Here's how the part is built. I have some questions about the finished solid (model axes, mm). A direction names the side the tool comes from. Round coordinates to 2 decimals unless told otherwise and drop trailing zeros. Order: outer loops, then holes, each group sorted by start corner. A loop starts at its lowest first (then second) coordinate and runs counter-clockwise, first axis right, second up. Notation, with made-up numbers: (-9.75, 47.25) - (10.25, 47.25) arc R29 ccw to (10.25, 85.25) - close; hole circle Ø3 at (-35, 14). An arc over 180 degrees is marked (long way). One line per item, written item: value.
from build123d import *

# Parameters (mm, degrees)
SKETCH1_W               = 40
SKETCH1_H               = 20
BOSS_EXTRUDE1_DEPTH     = 40
BOSS_EXTRUDE2_START     = -13.2
SKETCH2_W               = 55
SKETCH2_H               = 20
BOSS_EXTRUDE2_DEPTH     = 3.15
CUT_EXTRUDE1_DEPTH      = 42.871858091
CUT_EXTRUDE1_DEPTH_BACK = 42.871858091
SKETCH4_R               = 2.265
SKETCH5_R               = 6.5
BOSS_EXTRUDE3_DEPTH     = 1
SKETCH7_R               = 2.9
BOSS_EXTRUDE4_DEPTH     = 3.5
SKETCH8_W               = 6.5
SKETCH8_H               = 3.2
BOSS_EXTRUDE5_DEPTH     = 3


with BuildPart() as part:
    # Sketch1 → Boss-Extrude1 (new body)
    with BuildSketch(Plane(origin=(0, 0, 0), x_dir=(1, 0, 0), z_dir=(0, 1, 0))):
        Rectangle(SKETCH1_W, SKETCH1_H)
    extrude(amount=BOSS_EXTRUDE1_DEPTH)

    # Sketch2 → Boss-Extrude2 (add)
    with BuildSketch(Plane(origin=(0, 40, 0), x_dir=(1, 0, 0), z_dir=(0, 1, 0)).offset(BOSS_EXTRUDE2_START)):
        Rectangle(SKETCH2_W, SKETCH2_H)
    extrude(amount=BOSS_EXTRUDE2_DEPTH)

    # Sketch4 → Cut-Extrude1 (cut, two sides: drawn at the far end of the back side and taken through both)
    with BuildSketch(Plane(origin=(0, 29.95, 0), x_dir=(1, 0, 0), z_dir=(0, 1, 0)).offset(-CUT_EXTRUDE1_DEPTH_BACK)):
        with Locations(Location((-24.265, 5.005, 0), (0, 0, 270))):
            Circle(SKETCH4_R)
        with Locations(Location((-24.265, -5.005, 0), (0, 0, 270))):
            Circle(SKETCH4_R)
        with Locations(Location((24.265, -5.005, 0), (0, 0, 270))):
            Circle(SKETCH4_R)
        with Locations(Location((24.265, 5.005, 0), (0, 0, 270))):
            Circle(SKETCH4_R)
    extrude(amount=CUT_EXTRUDE1_DEPTH + CUT_EXTRUDE1_DEPTH_BACK, mode=Mode.SUBTRACT)

    # Sketch5 → Boss-Extrude3 (add)
    with BuildSketch(Plane(origin=(0, 40, 0), x_dir=(1, 0, 0), z_dir=(0, 1, 0))):
        with Locations(Location((10.5, 0, 0), (0, 0, 270))):
            Circle(SKETCH5_R)
    extrude(amount=BOSS_EXTRUDE3_DEPTH)

    # Sketch7 → Boss-Extrude4 (add)
    with BuildSketch(Plane(origin=(0, 41, 0), x_dir=(1, 0, 0), z_dir=(0, 1, 0))):
        with Locations(Location((10.5, 0, 0), (0, 0, 270))):
            Circle(SKETCH7_R)
    extrude(amount=BOSS_EXTRUDE4_DEPTH)

    # Sketch8 → Boss-Extrude5 (add)
    with BuildSketch(Plane(origin=(20, 0, 0), x_dir=(0, 0, -1), z_dir=(1, 0, 0))):
        with Locations((0, 4.9)):
            Rectangle(SKETCH8_W, SKETCH8_H)
    extrude(amount=BOSS_EXTRUDE5_DEPTH)


solid = part.part
Q1. If we section it at A-A, the plane z = 8.25: Please give me the cut outline in (x, y).
Results list:
outline: (-27.5, 26.8) - (-20, 26.8) - (-20, 0) - (20, 0) - (20, 26.8) - (27.5, 26.8) - (27.5, 29.95) - (20, 29.95) - (20, 40) - (-20, 40) - (-20, 29.95) - (-27.5, 29.95) - close
Q2. If we section it at D-D, the plane z = 0: Please give me the cut outline in (x, y), then the cut area to 3 significant figures.
Results list:
outline: (-27.5, 26.8) - (-20, 26.8) - (-20, 0) - (20, 0) - (20, 3.3) - (23, 3.3) - (23, 6.5) - (20, 6.5) - (20, 26.8) - (27.5, 26.8) - (27.5, 29.95) - (20, 29.95) - (20, 40) - (17, 40) - (17, 41) - (13.4, 41) - (13.4, 44.5) - (7.6, 44.5) - (7.6, 41) - (4, 41) - (4, 40) - (-20, 40) - (-20, 29.95) - (-27.5, 29.95) - close
area: 1,690 mm²
Q3. If we section it at B-B, the plane x = 10.5: Please give me the cut outline in (y, z).
Results list:
outline: (0, -10) - (40, -10) - (40, -6.5) - (41, -6.5) - (41, -2.9) - (44.5, -2.9) - (44.5, 2.9) - (41, 2.9) - (41, 6.5) - (40, 6.5) - (40, 10) - (0, 10) - close
Q4. Which directions (+Z, -Z, +X, -X, +Y, -Y) give clear straight access to the entire face, cutting with the end or side of a thin tool? Please do faces 1 (the flat face through (21, 5, -3.25)), 2 (the flat face through (-24, 26.8, 0)), 3 (the flat face through (9, 41, 3)), 4 (the flat face through (21, 5, 3.25)).
Results list:
face 1: -Z, +X, -Y
face 2: +Z, -Z, -X, -Y
face 3: +Y
face 4: +Z, +X, -Y
Q5. We'd pull the mould along Z, two halves only. Please class faces 5 (the flat face through (27.5, 28, 0)), 6 (the cylindrical face through (-22, 28, -5)), 7 (the cylindrical face through (16.945, 40.493, -0.846)), 8 (the cylindrical face through (22.9, 28.4, 3.2)): released by +Z, released by -Z, zero draft, split by the parting line, or undercut.
Results list:
face 5: zero draft
face 6: undercut
face 7: split by the parting line
face 8: undercut
Q6. Will these pins go through, and if not, where does the flat tip stop? pin 1 (2 mm diameter, centred on x = 24.5, z = 4, fed in from -Y); pin 2 (2.5 mm diameter, centred on x = 22, y = 5, fed in from -Z); pin 3 (0.9 mm diameter, centred on x = 21, z = -0.5, fed in from -Y); pin 4 (10 mm diameter, centred on x = -4.5, z = 5.5, fed in from +Y).
Results list:
pin 1: through
pin 2: z = -3.25
pin 3: y = 3.3
pin 4: y = 40
Q7. If I drill on line 1 along Y through (x, z) = (-20.5, -2.5); line 2 along Y through (x, z) = (-13.5, 4); line 3 along X through (y, z) = (7.5, -6.75), over which ranges is the centre line in solid material (lowest first)?
Results list:
line 1: 26.8 to 29.95
line 2: 0 to 40
line 3: -20 to 20
Q8. If we section it at C-C, the plane y = 38: Please give me the cut outline in (x, z), then the cut area to 3 significant figures.
Results list:
outline: (-20, -10) - (20, -10) - (20, 10) - (-20, 10) - close
area: 800 mm²
